Autodesk Inventor part; units mm, degrees
ref_plane "YZ Plane" through (0, 0, 0) normal (1, 0, 0) x (0, 1, 0)
ref_plane "XZ Plane" through (0, 0, 0) normal (0, 1, 0) x (-1, 0, 0)
ref_plane "XY Plane" through (0, 0, 0) normal (0, 0, 1) x (1, 0, 0)
sketch "Sketch1" plane through (0, 0, 0) normal (0, 1, 0) x (-1, 0, 0)
  circle A0 centre (0, 0) radius 1.5875
  dimension "d0" = 3.175
extrude "Extrusion1" add sketch "Sketch1" along normal blind 254
sketch "Sketch9" plane through (0, 0, 0) normal (1, 0, 0) x (0, 1, 0)
  line L0 (0, -1.5875) -> (0, 1.5875)
  line L1 (254, -1.5875) -> (254, 1.5875)
  line L2 (254, 0) -> (228.6, 0)
  line L3 (0, 0) -> (25.4, 0)
  dimension "d42" = 25.4
  dimension "d43" = 25.4
hole "Hole5" at (0, 25.4, 0) direction (-1, 0, 0) diameter 1.1906 end through all both
hole "Hole6" [suppressed]
sketch "Sketch10" plane through (0, 254, 0) normal (0, 1, 0) x (1, 0, 0)
  circle A0 centre (0, 0) radius 1.5875
hole "Hole7" at (0, 254, 0) direction (0, -1, 0) diameter 1.905 end through all
thread "Thread28"
thread "Thread29"
thread "Thread30"
thread "Thread31"
thread "Thread32"
thread "Thread33"
thread "Thread34"
thread "Thread35"
thread "Thread36"
thread "Thread37"
thread "Thread38"
thread "Thread40"
thread "Thread41"
thread "Thread42"
thread "Thread43"
thread "Thread44"
thread "Thread45"
thread "Thread46"
sketch "Sketch15" plane through (0, 254, 0) normal (0, 1, 0) x (1, 0, 0)
  circle A0 centre (0, 0) radius 1.5875
  circle A1 centre (0, 0) radius 0.9525
extrude "Extrusion4" cut sketch "Sketch15" against normal blind 86.36
properties part number "burder_rod_2"
CAD build for the part. Positions are in the model's coordinates, mm. Coordinates: 2 decimals unless noted, no trailing zeros. Order: outer loops, then holes, each group sorted by start corner. A loop starts at its lowest first (then second) coordinate and runs counter-clockwise, first axis right, second up.
Item 1: Band-saw the part on B-B on y = 158. List the corners of the cut face in (x, z) (1 decimal).
Check sheet entries:
outline: circle Ø3.2 at (0, 0); hole circle Ø1.9 at (0, 0)
Item 2: Drill centre lines: L1, parallel to Y at x = 1.35, z = 0; L2, parallel to X at y = 124.5, z = 0.15; L3, parallel to Z at x = 0, y = 90. Where is each one in solid material? Low to high.
Check sheet entries:
L1: y = 0 to 24.8, 26 to 167.64
L2: x = -1.58 to -0.94, 0.94 to 1.58
L3: z = -1.59 to -0.95, 0.95 to 1.59
Item 3: Band-saw the part on A-A on x = 0. List the corners of the cut face in (y, z).
Check sheet entries:
outline: (0, -1.59) - (167.64, -1.59) - (167.64, -0.95) - (0, -0.95) - close; (0, 0.95) - (167.64, 0.95) - (167.64, 1.59) - (0, 1.59) - close
Item 4: Pin check, flat tips, straight feed: pin 1 Ø1 at (x, y) = (-1, 138.5) entering from +Z; pin 2 Ø1.1 at (y, z) = (25.4, 0) entering from -X. Stop position of each tip, or through.
Check sheet entries:
pin 1: stops at z = 1.51
pin 2: passes through
